Answer from the drawing. Dimensions are ordinates in mm from the lowest x, y and z of the part. A direction names the side the tool comes from. Round coordinates to 2 decimals unless told otherwise and drop trailing zeros. Write each loop counter-clockwise with the first axis right and the second up, starting at its lowest first coordinate (ties: lowest second). Pieces come first, ordered by that corner, then holes.
1. Find section C-C (x = 3.25). Write down the section's boundary in (y, z), and give its area (3 significant figures).
2. Find section D-D (y = 1). Write down the section's boundary in (x, z).
3. A tool of negligible diameter and unlimited length cuts with its end or side. For the marked faces 5 and 6, from which of +Z, -Z, +X, -X, +Y, -Y can it reach the whole face along a straight path? Write none if from no direction.
4. Find section B-B (z = 7.25). Write down the section's boundary in (x, y), and give its area (3 significant figures).
5. Find section A-A (y = 7.5). Write down the section's boundary in (x, z).
6. Determine the mould class of the marked faces 1, 2, 3 and 4 for opening direction Y: pulls with the +Y half, pulls with the -Y half, needs draft (parallel to the pull), parting line crosses it, or undercut.
7. Straight lines are drawn through the part: probe 1 along Y at (x, z) = (7.5, 1.35); probe 2 along X at (y, z) = (8, 9.5); probe 3 along Z at (x, y) = (9, 2.5). For each, find the intervals that lie inside material, in ascending order.
8. A flat-ended cylindrical pin translates along its axis: pin 1 Ø3 at (y, z) = (9.5, 7.5) entering from -X. Find the tip coordinate at first contact, or state that the pin passes through.
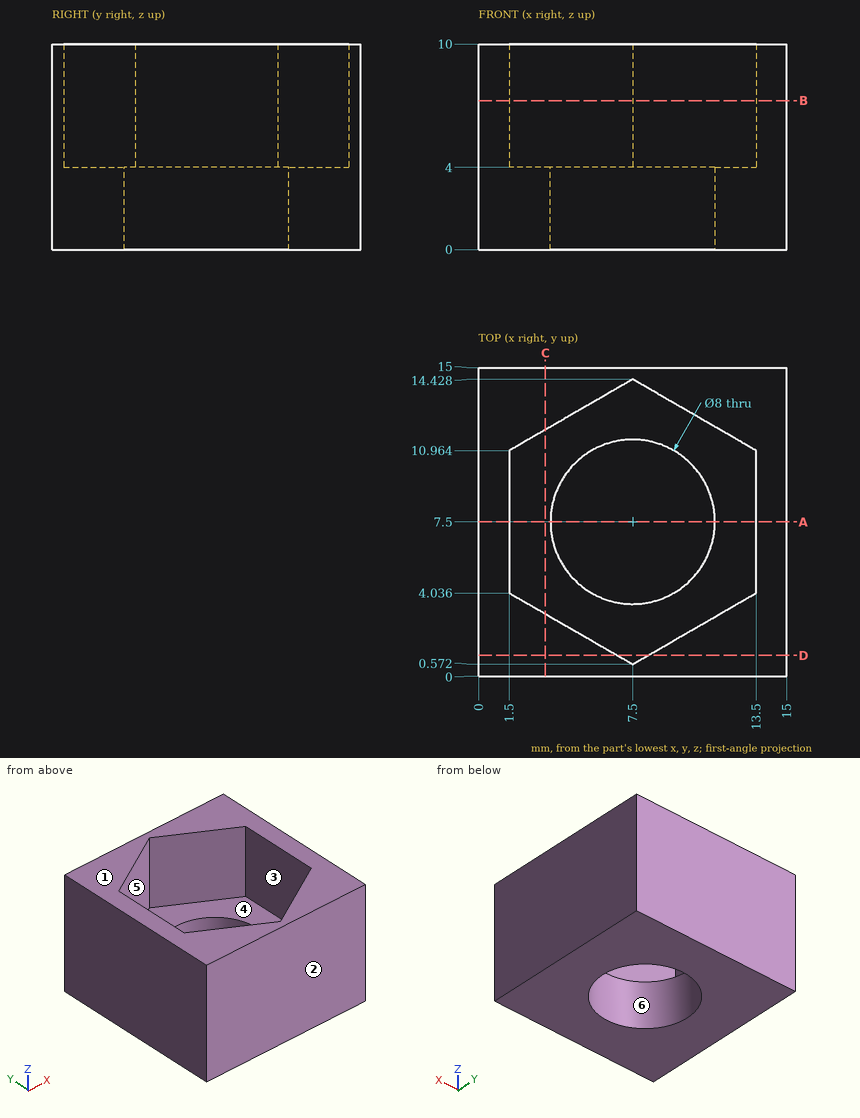
Worked answers:
1. outline: (0, 0) - (15, 0) - (15, 10) - (11.97, 10) - (11.97, 4) - (3.03, 4) - (3.03, 10) - (0, 10) - close
1. area: 96.3 mm2
2. outline: (0, 0) - (15, 0) - (15, 10) - (8.24, 10) - (8.24, 4) - (6.76, 4) - (6.76, 10) - (0, 10) - close
3. face 5: +Z
3. face 6: +Z, -Z
4. outline: (0, 0) - (15, 0) - (15, 15) - (0, 15) - close; hole (1.5, 4.04) - (7.5, 0.57) - (13.5, 4.04) - (13.5, 10.96) - (7.5, 14.43) - (1.5, 10.96) - close
4. area: 100 mm2
5. outline: (0, 0) - (3.5, 0) - (3.5, 4) - (1.5, 4) - (1.5, 10) - (0, 10) - close; (11.5, 0) - (15, 0) - (15, 10) - (13.5, 10) - (13.5, 4) - (11.5, 4) - close
6. face 1: needs draft
6. face 2: pulls with the -Y half
6. face 3: undercut
6. face 4: undercut
7. probe 1: y = 0 to 3.5, 11.5 to 15
7. probe 2: x = 0 to 1.5, 13.5 to 15
7. probe 3: z = 0 to 4
8. pin 1: stops at x = 0
